```python
from build123d import *

# Parameters (mm, degrees)
BOSS_EXTRUDE1_DEPTH     = 77.5
SKETCH2_W               = 45
SKETCH2_H               = 45
BOSS_EXTRUDE2_DEPTH     = 2.5
CUT_EXTRUDE1_DEPTH      = 93.478375851
CUT_EXTRUDE1_DEPTH_BACK = 93.478375851
SKETCH3_R               = 1.5
CHAMFER3_SIZE           = 1.5
CHAMFER2_SIZE           = 1
FILLET1_R               = 1.5


with BuildPart() as part:
    # Sketch1 → Boss-Extrude1 (new body)
    with BuildSketch(Plane(origin=(0, 0, 0), x_dir=(1, 0, 0), z_dir=(0, 1, 0))):
        Polygon((-11, 2.116025404), (-11, -2.116025404), (-12.5, -1.25), (-12.5, -12.5), (-1, -12.5), (-1.866025404, -14), (1.866025404, -14), (1, -12.5), (12.5, -12.5), (24, -12.5), (23.133974596, -14), (26.866025404, -14), (26, -12.5), (37.5, -12.5), (37.5, -1), (39, -1.866025404), (39, 1.866025404), (37.5, 1), (37.5, 12.5), (37.5, 24), (39, 23.133974596), (39, 26.866025404), (37.5, 26), (37.5, 37.5), (26.25, 37.5), (27.116025404, 36), (22.883974596, 36), (23.75, 37.5), (12.5, 37.5), (1.25, 37.5), (2.116025404, 36), (-2.116025404, 36), (-1.25, 37.5), (-12.5, 37.5), (-12.5, 26.25), (-11, 27.116025404), (-11, 22.883974596), (-12.5, 23.75), (-12.5, 12.5), (-12.5, 1.25), align=None)
        Polygon((-10, 10), (-10, -10), (10, -10), (15, -10), (35, -10), (35, 10), (35, 15), (35, 35), (15, 35), (10, 35), (-10, 35), (-10, 15), align=None, mode=Mode.SUBTRACT)
    extrude(amount=BOSS_EXTRUDE1_DEPTH)

    # Sketch2 → Boss-Extrude2 (add)
    with BuildSketch(Plane(origin=(0, 0, 0), x_dir=(1, 0, 0), z_dir=(0, 1, 0))):
        with Locations((12.5, 12.5)):
            Rectangle(SKETCH2_W, SKETCH2_H)
    extrude(amount=BOSS_EXTRUDE2_DEPTH)

    # Sketch3 → Cut-Extrude1 (cut, two sides: drawn at the far end of the back side and taken through both)
    with BuildSketch(Plane(origin=(0, 2.5, 0), x_dir=(1, 0, 0), z_dir=(0, 1, 0)).offset(-CUT_EXTRUDE1_DEPTH_BACK)):
        with Locations(Location((-6, 6, 0), (0, 0, 270))):
            Circle(SKETCH3_R)
        with Locations(Location((6, 6, 0), (0, 0, 270))):
            Circle(SKETCH3_R)
        with Locations(Location((6, -6, 0), (0, 0, 270))):
            Circle(SKETCH3_R)
        with Locations(Location((-6, -6, 0), (0, 0, 270))):
            Circle(SKETCH3_R)
        with Locations(Location((31, -6, 0), (0, 0, 270))):
            Circle(SKETCH3_R)
        with Locations(Location((19, -6, 0), (0, 0, 270))):
            Circle(SKETCH3_R)
        with Locations(Location((19, 6, 0), (0, 0, 270))):
            Circle(SKETCH3_R)
        with Locations(Location((31, 6, 0), (0, 0, 270))):
            Circle(SKETCH3_R)
        with Locations(Location((31, 19, 0), (0, 0, 270))):
            Circle(SKETCH3_R)
        with Locations(Location((19, 19, 0), (0, 0, 270))):
            Circle(SKETCH3_R)
        with Locations(Location((19, 31, 0), (0, 0, 270))):
            Circle(SKETCH3_R)
        with Locations(Location((31, 31, 0), (0, 0, 270))):
            Circle(SKETCH3_R)
        with Locations(Location((-6, 31, 0), (0, 0, 270))):
            Circle(SKETCH3_R)
        with Locations(Location((6, 31, 0), (0, 0, 270))):
            Circle(SKETCH3_R)
        with Locations(Location((6, 19, 0), (0, 0, 270))):
            Circle(SKETCH3_R)
        with Locations(Location((-6, 19, 0), (0, 0, 270))):
            Circle(SKETCH3_R)
    extrude(amount=CUT_EXTRUDE1_DEPTH + CUT_EXTRUDE1_DEPTH_BACK, mode=Mode.SUBTRACT)

    # Chamfer3
    chamfer3_edges = [part.edges().sort_by_distance(p)[0] for p in [
        (39, 0, -25),
        (0, 0, 14),
        (25, 0, 14),
        (39, 0, 0),
        (-11, 0, 0),
        (-11, 0, -25),
        (0, 0, -36),
        (25, 0, -36),
        (-12.5, 0, -12.5),
        (-12.5, 0, 6.875),
        (-6.75, 0, 12.5),
        (12.5, 0, 12.5),
        (31.75, 0, 12.5),
        (37.5, 0, 6.75),
        (37.5, 0, -12.5),
        (-12.5, 0, -31.875),
        (-6.875, 0, -37.5),
        (12.5, 0, -37.5),
        (37.5, 0, -31.75),
        (31.875, 0, -37.5),
    ]]
    chamfer(chamfer3_edges, length=CHAMFER3_SIZE - 0.0001)  # a hair under: the kernel refuses the full size

    # Chamfer2
    chamfer2_edges = [part.edges().sort_by_distance(p)[0] for p in [
        (12.5, 2.5, -35),
        (-10, 2.5, -12.5),
        (12.5, 2.5, 10),
        (35, 2.5, -12.5),
        (31, 2.5, -20.5),
        (31, 2.5, -7.5),
        (19, 2.5, -7.5),
        (19, 2.5, 4.5),
        (6, 2.5, -7.5),
        (6, 2.5, 4.5),
        (-6, 2.5, 4.5),
        (31, 2.5, 4.5),
        (-6, 2.5, -20.5),
        (6, 2.5, -20.5),
        (6, 2.5, -32.5),
        (19, 2.5, -20.5),
        (19, 2.5, -32.5),
        (31, 2.5, -32.5),
        (-6, 2.5, -32.5),
        (-6, 2.5, -7.5),
    ]]
    chamfer(chamfer2_edges, length=CHAMFER2_SIZE)

    # Fillet1
    fillet1_edges = [part.edges().sort_by_distance(p)[0] for p in [
        (35, 40.5, -35),
        (-10, 40.5, -35),
        (-10, 40.5, 10),
        (35, 40.5, 10),
    ]]
    fillet(fillet1_edges, radius=FILLET1_R)


solid = part.part
```
For this review, take the finished solid that the model builds, in its own axes (mm). Round coordinates to 2 decimals unless told otherwise and drop trailing zeros. Write each loop counter-clockwise with the first axis right and the second up, starting at its lowest first coordinate (ties: lowest second). Pieces come first, ordered by that corner, then holes.
1) Take a section at A-A on z = -10. Give the boundary of the cut face in (x, y).
Answer below:
outline: (-12.5, 1.5) - (-11, 0) - (36, 0) - (37.5, 1.5) - (37.5, 77.5) - (35, 77.5) - (35, 3.5) - (34, 2.5) - (-9, 2.5) - (-10, 3.5) - (-10, 77.5) - (-12.5, 77.5) - close
2) Take a section at C-C on z = -31. State how many separate pieces and enclosed holes the cut face has, then the cut area to 3 significant figures.
Answer below:
separate pieces: 5
enclosed holes: 0
area: 465 mm2
3) Insertion check: pin 1 Ø4 at (x, z) = (19, -31) entering from +Y; pin 2 Ø12 at (x, z) = (12.5, -24) entering from +Y; pin 3 Ø3.5 at (x, z) = (-6, -31) entering from +Y. Each pin has a flat end and moves straight along its axis. Give the tip position at first contact, or say it passes through.
Answer below:
pin 1: stops at y = 2
pin 2: stops at y = 2.5
pin 3: stops at y = 1.75
4) For line 1 along Z through (x, y) = (17, 7); line 2 along X through (y, z) = (31.5, -21); line 3 along Z through (x, y) = (31, 1), list the stretches that pass through material, from the lowest coordinate up.
Answer below:
line 1: z = -37.5 to -35, 10 to 12.5
line 2: x = -12.5 to -10, 35 to 37.5
line 3: z = -37 to -32.5, -29.5 to -20.5, -17.5 to -7.5, -4.5 to 4.5, 7.5 to 12
5) Take a section at B-B on x = 12.5. Give the boundary of the cut face in (y, z).
Answer below:
outline: (0, -36) - (1.5, -37.5) - (77.5, -37.5) - (77.5, -35) - (3.5, -35) - (2.5, -34) - (2.5, 9) - (3.5, 10) - (77.5, 10) - (77.5, 12.5) - (1.5, 12.5) - (0, 11) - close
6) Mouldability with a two-part tool opening along X and no side actions: class faces 1 (the face through (-6, 2, -21)), 2 (the face through (33, 2, -31)), 3 (the face through (39, 39, 0)), 4 (the face through (13, 39, -37.5)) as +X half, -X half, draft (parallel to the pull), parting line (faces both ways), or undercut.
Answer below:
face 1: undercut
face 2: undercut
face 3: +X half
face 4: draft
